```python
from build123d import *

# Parameters (mm, degrees)
SKETCH1_R           = 7.8
SKETCH1_R_2         = 2.5
SKETCH1_R_3         = 1.4
BOSS_EXTRUDE1_DEPTH = 4.5


with BuildPart() as part:
    # Sketch1 → Boss-Extrude1 (new body)
    with BuildSketch(Plane.XY):
        with BuildLine():
            Line((-8.991382593, -0.39375), (-12.488031379, 79.453125))
            ThreePointArc((-12.488031379, 79.453125), (0, 92.5), (12.488031379, 79.453125))
            Line((12.488031379, 79.453125), (8.991382593, -0.39375))
            ThreePointArc((8.991382593, -0.39375), (0, -9), (-8.991382593, -0.39375))
        make_face()
        with Locations((0, 80)):
            Circle(SKETCH1_R, mode=Mode.SUBTRACT)
        Circle(SKETCH1_R_2, mode=Mode.SUBTRACT)
        with Locations((0, 5.5)):
            Circle(SKETCH1_R_3, mode=Mode.SUBTRACT)
        with Locations((0, -5.5)):
            Circle(SKETCH1_R_3, mode=Mode.SUBTRACT)
    extrude(amount=BOSS_EXTRUDE1_DEPTH)


solid = part.part
```
The model under review builds one solid part; all positions refer to its coordinate system, in mm. Give positions to 0.01 mm unless a question says otherwise; leave off trailing zeros. Write each loop counter-clockwise with the first axis right and the second up, starting at its lowest first coordinate (ties: lowest second). Pieces come first, ordered by that corner, then holes. Notation, with made-up numbers: M 79.25,13.5 L 93.25,13.5 A18 ccw 93.25,19.5 Z; hole C 20,83.25 d7. An arc over 180 degrees is marked long. Write item = value, one per line. Start each with the question number.
Q1. We need section B-B (z = 1.55). State the section outline as (x, y) points.
Q2. For line 1 (Y direction, x = -0.5, z = 3.6); line 2 (Y direction, x = 2.75, z = 1.05); line 3 (Y direction, x = 6.5, z = 1.3), list the stretches that pass through material, from the lowest coordinate up.
Q3. Mouldability with a two-part tool opening along Y and no side actions: class faces 1 (the face through (0, 42, 4.5)), 2 (the face through (-0.18, 6.89, 2.22)), 3 (the face through (-10.715, 38.971, 2.218)) as released by +Y, released by -Y, zero draft, split by the parting line, or undercut.
Q4. We need section C-C (y = -5.5). State the section outline as (x, z) points, plus the area to 3 significant figures.
Q5. We need section D-D (y = 5.5). State the section outline as (x, z) points.
Q6. Clearance check with flat-ended pins moving along their axes: pin 1 (1.7 mm diameter, centred on x = 0, y = -5.5, fed in from +Z); pin 2 (1 mm diameter, centred on y = 76.5, z = 2, fed in from +X); pin 3 (2 mm diameter, centred on x = 8.5, z = 2.5, fed in from +Y); pin 4 (2 mm diameter, centred on x = 3, z = 4, fed in from +Y). State where each tip first meets the part, or that it passes through.
Q7. We need section A-A (x = 0). State the section outline as (y, z) points, plus the area to 3 significant figures.
Result set:
q1.outline = M -12.49,79.45 L -8.99,-0.39 A9 ccw 8.99,-0.39 L 12.49,79.45 A12.5 ccw long Z; hole C 0,80 d15.6; hole C 0,0 d5; hole C 0,-5.5 d2.8; hole C 0,5.5 d2.8
q2.line_1 = -8.99 to -6.81, -4.19 to -2.45, 2.45 to 4.19, 6.81 to 72.22, 87.78 to 92.49
q2.line_2 = -8.57 to 72.7, 87.3 to 92.19
q2.line_3 = -6.22 to 75.69, 84.31 to 90.68
q3.face_1 = zero draft
q3.face_2 = undercut
q3.face_3 = released by -Y
q4.outline = M -7.12,0 L -1.4,0 L -1.4,4.5 L -7.12,4.5 Z; M 1.4,0 L 7.12,0 L 7.12,4.5 L 1.4,4.5 Z
q4.area = 51.5 mm2
q5.outline = M -9.25,0 L -1.4,0 L -1.4,4.5 L -9.25,4.5 Z; M 1.4,0 L 9.25,0 L 9.25,4.5 L 1.4,4.5 Z
q6.pin_1 = through
q6.pin_2 = 12.38
q6.pin_3 = 90
q6.pin_4 = 92.34
q7.outline = M -9,0 L -6.9,0 L -6.9,4.5 L -9,4.5 Z; M -4.1,0 L -2.5,0 L -2.5,4.5 L -4.1,4.5 Z; M 2.5,0 L 4.1,0 L 4.1,4.5 L 2.5,4.5 Z; M 6.9,0 L 72.2,0 L 72.2,4.5 L 6.9,4.5 Z; M 87.8,0 L 92.5,0 L 92.5,4.5 L 87.8,4.5 Z
q7.area = 339 mm2
